The model under review builds one solid part; all positions refer to its coordinate system, in mm. A direction names the side the tool comes from. Coordinates: 2 decimals unless noted, no trailing zeros. Order: outer loops, then holes, each group sorted by start corner. A loop starts at its lowest first (then second) coordinate and runs counter-clockwise, first axis right, second up. Notation, with made-up numbers: (44, -7) -> (97, -7) arc R19 cw to (97, 20) -> close; hole circle Ø4 at (44, -20). An arc over 180 degrees is marked (long way). Use one line per item in the form item = value. Start each with the question number.
(1) Take a section at C-C (x = 3.75). State the section outline as (y, z) points (3 decimals).
(2) Insertion check: pin 1 Ø5.5 at (x, z) = (11.5, -4) entering from -Y. The pin has a flat end and moves straight along its axis. Give the tip position at first contact, or say it passes through.
(3) Take a section at B-B (z = -1.5). State the section outline as (x, y) points (3 decimals), then the cut area to 3 significant figures.
(4) Take a section at A-A (y = 0.6). State how many separate pieces and enclosed holes the cut face has, then the cut area to 3 significant figures.
(5) Wall thickness on line 1 along X through (y, z) = (1, -2.5) (3 decimals); line 2 along Z through (x, y) = (5.75, 1.15) (3 decimals); line 3 along Z through (x, y) = (10, 0.15) (3 decimals): over which ranges is each line inside the solid? List them lowest first.
(6) Take a section at D-D (z = -6.35). State the section outline as (x, y) points (1 decimal).
(7) For faces 1 (the flat face through (0, 1, -6)), 2 (the flat face through (21.59, 1, -6)), list the 3-axis set-ups (+Z, -Z, +X, -X, +Y, -Y) from which the entire face can be reached by the end or side of a thin tool; tool diameter is ignored.
(8) Mouldability with a two-part tool opening along X and no side actions: class faces 3 (the flat face through (22.225, 1, -6)), 4 (the flat face through (8.6, 1.905, -7.7)), 5 (the flat face through (11, 0, -6)), 6 (the flat face through (0.635, 1, -6)) as +X half, -X half, draft (parallel to the pull), parting line (faces both ways), or undercut.
```python
from build123d import *

# Parameters (mm, degrees)
SKETCH1_W           = 22.225
SKETCH1_H           = 12.7
BOSS_EXTRUDE1_DEPTH = 2.54
FILLET1_R           = 0.635
SHELL1_START        = 0.635
SHELL1_OUTLINE_W    = 1.905
SHELL1_OUTLINE_H    = 11.43
SHELL1_DEPTH        = 20.955
SKETCH2_R           = 2.54
BOSS_EXTRUDE2_DEPTH = 1.905


# Read off the part's stored shape, not the designer's step: Shell1
with BuildPart() as part:
    # Sketch1 → Boss-Extrude1 (new body)
    with BuildSketch(Plane(origin=(0, 0, 0), x_dir=(1, 0, 0), z_dir=(0, 1, 0))):
        with Locations((11.1125, 6.35)):
            Rectangle(SKETCH1_W, SKETCH1_H)
    extrude(amount=BOSS_EXTRUDE1_DEPTH)

    # Fillet1
    fillet1_edges = [part.edges().sort_by_distance(p)[0] for p in [
        (0, 1.27, -12.7),
        (22.225, 1.27, -12.7),
        (22.225, 1.27, 0),
        (0, 1.27, 0),
    ]]
    fillet(fillet1_edges, radius=FILLET1_R)

    # Shell1 outline → Shell1 (cut)
    with BuildSketch(Plane.YZ.offset(SHELL1_START)):
        with Locations((0.9525, -6.35)):
            Rectangle(SHELL1_OUTLINE_W, SHELL1_OUTLINE_H)
    extrude(amount=SHELL1_DEPTH, mode=Mode.SUBTRACT)

    # Sketch2 → Boss-Extrude2 (add)
    with BuildSketch(Plane(origin=(0, 1.905, 0), x_dir=(-1, 0, 0), z_dir=(0, -1, 0))):
        with Locations(Location((-11.1125, 6.35, 0), (0, 0, 270))):
            Circle(SKETCH2_R)
    extrude(amount=BOSS_EXTRUDE2_DEPTH)


solid = part.part
```
Findings:
q1.outline = (0, -12.7) -> (2.54, -12.7) -> (2.54, 0) -> (0, 0) -> (0, -0.635) -> (1.905, -0.635) -> (1.905, -12.065) -> (0, -12.065) -> close
q2.pin_1 = 0
q3.outline = (0, 0) -> (0.635, 0) -> (0.635, 1.905) -> (21.59, 1.905) -> (21.59, 0) -> (22.225, 0) -> (22.225, 2.54) -> (0, 2.54) -> close
q3.area = 16.5 mm²
q4.separate_pieces = 2
q4.enclosed_holes = 1
q4.area = 62.7 mm²
q5.line_1 = 0 to 0.635, 21.59 to 22.225
q5.line_2 = -12.7 to -12.065, -0.635 to 0
q5.line_3 = -12.7 to -12.065, -8.633 to -4.067, -0.635 to 0
q6.outline = (0, 0) -> (0.6, 0) -> (0.6, 1.9) -> (8.6, 1.9) -> (8.6, 0) -> (13.7, 0) -> (13.7, 1.9) -> (21.6, 1.9) -> (21.6, 0) -> (22.2, 0) -> (22.2, 2.5) -> (0, 2.5) -> close
q7.face_1 = +Z, -Z, -X, +Y, -Y
q7.face_2 = -Y
q8.face_3 = +X half
q8.face_4 = undercut
q8.face_5 = draft
q8.face_6 = undercut
